```python
from build123d import *

# Parameters (mm, degrees)
BOSS_EXTRUDE1_DEPTH = 7
SKETCH2_W           = 10
SKETCH2_H           = 10
BOSS_EXTRUDE2_DEPTH = 95
SKETCH3_R           = 37.663730654
CUT_EXTRUDE1_DEPTH  = 130.030393965
CIRPATTERN1_COUNT   = 8


with BuildPart() as part:
    # Sketch1 → Boss-Extrude1 (new body)
    with BuildSketch(Plane(origin=(0, 0, 0), x_dir=(1, 0, 0), z_dir=(0, 1, 0))):
        with BuildLine():
            Line((-8, 56.940758688), (-8, 59.740758688))
            ThreePointArc((-8, 59.740758688), (-7.414213562, 61.154972251), (-6, 61.740758688))
            Line((-6, 61.740758688), (6, 61.740758688))
            ThreePointArc((6, 61.740758688), (7.414213562, 61.154972251), (8, 59.740758688))
            Line((8, 59.740758688), (8, 56.940758688))
            ThreePointArc((8, 56.940758688), (22.004297361, 53.123073119), (34.606342345, 45.920050844))
            Line((34.606342345, 45.920050844), (36.586241332, 47.899949831))
            ThreePointArc((36.586241332, 47.899949831), (38.000454895, 48.485736269), (39.414668457, 47.899949831))
            Line((39.414668457, 47.899949831), (47.899949831, 39.414668457))
            ThreePointArc((47.899949831, 39.414668457), (48.485736269, 38.000454895), (47.899949831, 36.586241332))
            Line((47.899949831, 36.586241332), (45.920050844, 34.606342345))
            ThreePointArc((45.920050844, 34.606342345), (53.123073119, 22.004297361), (56.940758688, 8))
            Line((56.940758688, 8), (59.740758688, 8))
            ThreePointArc((59.740758688, 8), (61.154972251, 7.414213562), (61.740758688, 6))
            Line((61.740758688, 6), (61.740758688, -6))
            ThreePointArc((61.740758688, -6), (61.154972251, -7.414213562), (59.740758688, -8))
            Line((59.740758688, -8), (56.940758688, -8))
            ThreePointArc((56.940758688, -8), (53.123073119, -22.004297361), (45.920050844, -34.606342345))
            Line((45.920050844, -34.606342345), (47.899949831, -36.586241332))
            ThreePointArc((47.899949831, -36.586241332), (48.485736269, -38.000454895), (47.899949831, -39.414668457))
            Line((47.899949831, -39.414668457), (39.414668457, -47.899949831))
            ThreePointArc((39.414668457, -47.899949831), (38.000454895, -48.485736269), (36.586241332, -47.899949831))
            Line((36.586241332, -47.899949831), (34.606342345, -45.920050844))
            ThreePointArc((34.606342345, -45.920050844), (22.004297361, -53.123073119), (8, -56.940758688))
            Line((8, -56.940758688), (8, -59.740758688))
            ThreePointArc((8, -59.740758688), (7.414213562, -61.154972251), (6, -61.740758688))
            Line((6, -61.740758688), (-6, -61.740758688))
            ThreePointArc((-6, -61.740758688), (-7.414213562, -61.154972251), (-8, -59.740758688))
            Line((-8, -59.740758688), (-8, -56.940758688))
            ThreePointArc((-8, -56.940758688), (-22.004297361, -53.123073119), (-34.606342345, -45.920050844))
            Line((-34.606342345, -45.920050844), (-36.586241332, -47.899949831))
            ThreePointArc((-36.586241332, -47.899949831), (-38.000454895, -48.485736269), (-39.414668457, -47.899949831))
            Line((-39.414668457, -47.899949831), (-47.899949831, -39.414668457))
            ThreePointArc((-47.899949831, -39.414668457), (-48.485736269, -38.000454895), (-47.899949831, -36.586241332))
            Line((-47.899949831, -36.586241332), (-45.920050844, -34.606342345))
            ThreePointArc((-45.920050844, -34.606342345), (-53.123073119, -22.004297361), (-56.940758688, -8))
            Line((-56.940758688, -8), (-59.740758688, -8))
            ThreePointArc((-59.740758688, -8), (-61.154972251, -7.414213562), (-61.740758688, -6))
            Line((-61.740758688, -6), (-61.740758688, 6))
            ThreePointArc((-61.740758688, 6), (-61.154972251, 7.414213562), (-59.740758688, 8))
            Line((-59.740758688, 8), (-56.940758688, 8))
            ThreePointArc((-56.940758688, 8), (-53.123073119, 22.004297361), (-45.920050844, 34.606342345))
            Line((-45.920050844, 34.606342345), (-47.899949831, 36.586241332))
            ThreePointArc((-47.899949831, 36.586241332), (-48.485736269, 38.000454895), (-47.899949831, 39.414668457))
            Line((-47.899949831, 39.414668457), (-39.414668457, 47.899949831))
            ThreePointArc((-39.414668457, 47.899949831), (-38.000454895, 48.485736269), (-36.586241332, 47.899949831))
            Line((-36.586241332, 47.899949831), (-34.606342345, 45.920050844))
            ThreePointArc((-34.606342345, 45.920050844), (-22.004297361, 53.123073119), (-8, 56.940758688))
        make_face()
    extrude(amount=BOSS_EXTRUDE1_DEPTH)

    # Sketch2 → Boss-Extrude2 (add)
    with BuildSketch(Plane(origin=(0, 7, 0), x_dir=(1, 0, 0), z_dir=(0, 1, 0))):
        with Locations((45, 0)):
            Rectangle(SKETCH2_W, SKETCH2_H)
        with Locations((-45, 0)):
            Rectangle(SKETCH2_W, SKETCH2_H)
    extrude(amount=BOSS_EXTRUDE2_DEPTH)

    # Sketch3 → Cut-Extrude1 (cut, through all)
    with BuildSketch(Plane(origin=(0, 7, 0), x_dir=(1, 0, 0), z_dir=(0, 1, 0))):
        with Locations(Location((0, 0, 0), (0, 0, 270))):
            Circle(SKETCH3_R)
    extrude(amount=-CUT_EXTRUDE1_DEPTH, mode=Mode.SUBTRACT)

    # Sketch7 → Cut-Loft1 section 0
    with BuildSketch(Plane.XZ):
        with BuildLine():
            Line((-6, -57.040758688), (6, -57.040758688))
            Line((6, -57.040758688), (6, -59.340758688))
            Line((6, -59.340758688), (-6, -59.340758688))
            Line((-6, -59.340758688), (-6, -57.040758688))
        make_face()
    # Sketch5 → Cut-Loft1 section 1
    with BuildSketch(Plane(origin=(0, 7, 0), x_dir=(1, 0, 0), z_dir=(0, 1, 0))):
        with BuildLine():
            Line((-6, 59.740758688), (6, 59.740758688))
            Line((6, 59.740758688), (6, 57.040758688))
            Line((6, 57.040758688), (-6, 57.040758688))
            Line((-6, 57.040758688), (-6, 59.740758688))
        make_face()
    cut_loft1 = loft(mode=Mode.SUBTRACT)

    # CirPattern1: Cut-Loft1 ×8 about axis
    cirpattern1_axis = Axis((0, 0, 0), (0, 1, 0))
    for i in range(1, CIRPATTERN1_COUNT):
        add(cut_loft1.rotate(cirpattern1_axis, i * 360 / CIRPATTERN1_COUNT), mode=Mode.SUBTRACT)


solid = part.part
```
Input: part model. Units: mm. Frame: model coordinates. A direction names the side the tool comes from. Round coordinates to 2 decimals unless told otherwise and drop trailing zeros. Loops run counter-clockwise (first coordinate to the right, second up) from the corner with the lowest first, then second, coordinate; pieces in that order, holes last. Notation, with made-up numbers: (81, 50) - (86, 50) arc R23 ccw to (86, 87) - close; hole circle Ø5 at (3.25, 2). An arc over 180 degrees is marked (long way). One line per item, written item: value. Start each with the question number.
(1) Section C-C, the plane y = 27.5. Return loops of the section in (x, z).
(2) Contact query for flat-ended pins moving along their axis: P1, Ø5, axis at x = -44, y = 77, coming from the +Z side; P2, Ø0.8, axis at y = 5, z = -58.5, coming from the -X side; P3, Ø3, axis at x = -47, y = 51.5, coming from the -Z side. Output: stop coordinate, or through.
(3) Ray query, line 1 (X direction, y = 1.75, z = 0); line 2 (X direction, y = 2, z = 0); line 3 (Z direction, x = 46, y = 68.5). Return the intervals inside material, ascending. Write a range as [from, to].
(4) Section B-B, the plane z = 0. Return loops of the section in (x, y), plus the area to 3 significant figures.
(5) Section A-A, the plane x = 0. Return loops of the section in (y, z).
(6) Section D-D, the plane x = -17.5. Return loops of the section in (y, z), plus the area to 3 significant figures.
(7) Draft query along X for faces 1 (the flat face through (42.044, 3.549, 42.163)), 2 (the flat face through (0, 3, 61.741)), 3 (the flat face through (50, 54, 0)). Return one class per face: +X half, -X half, draft (parallel to the pull), parting line (faces both ways), or undercut.
(8) Access query for faces 4 (the flat face through (45, 54, 5)), 5 (the flat face through (59.544, 3.549, 0.084)), 6 (the flat face through (-40, 54, 0)), 7 (the flat face through (0, 4, 57.041)). Directions: +Z, -Z, +X, -X, +Y, -Y. A direction counts if a zero-diameter tool reaches every point of the face in a straight line with its end or side. Return the directions, or none.
Results below:
1. outline: (-50, -5) - (-40, -5) - (-40, 5) - (-50, 5) - close; (40, -5) - (50, -5) - (50, 5) - (40, 5) - close
2. P1: z = 5
2. P2: x = -8
2. P3: z = -5
3. line 1: [-61.74, -59.44], [-57.04, -37.66], [37.66, 57.04], [59.44, 61.74]
3. line 2: [-61.74, -59.46], [-57.04, -37.66], [37.66, 57.04], [59.46, 61.74]
3. line 3: [-5, 5]
4. outline: (-61.74, 0) - (-59.34, 0) - (-59.74, 7) - (-61.74, 7) - close; (-57.04, 0) - (-37.66, 0) - (-37.66, 7) - (-40, 7) - (-40, 102) - (-50, 102) - (-50, 7) - (-57.04, 7) - close; (37.66, 0) - (57.04, 0) - (57.04, 7) - (50, 7) - (50, 102) - (40, 102) - (40, 7) - (37.66, 7) - close; (59.34, 0) - (61.74, 0) - (61.74, 7) - (59.74, 7) - close
4. area: 2,200 mm^2
5. outline: (0, -61.74) - (7, -61.74) - (7, -59.74) - (0, -59.34) - close; (0, -57.04) - (7, -57.04) - (7, -37.66) - (0, -37.66) - close; (0, 37.66) - (7, 37.66) - (7, 57.04) - (0, 57.04) - close; (0, 59.34) - (7, 59.74) - (7, 61.74) - (0, 61.74) - close
6. outline: (0, -54.77) - (7, -54.77) - (7, -33.35) - (0, -33.35) - close; (0, 33.35) - (7, 33.35) - (7, 54.77) - (0, 54.77) - close
6. area: 300 mm^2
7. face 1: undercut
7. face 2: draft
7. face 3: +X half
8. face 4: +Z, +X, -X, +Y
8. face 5: +Y
8. face 6: +Z, -Z, +Y
8. face 7: +Y, -Y
